```python
from build123d import *

# Parameters (mm, degrees)
F1_DEPTH = 1587.5
F2_R     = 3.175
F3_DEPTH = 25.401
F4_W     = 25.4
F4_H     = 393.7
F5_DEPTH = 3.175


with BuildPart() as f1:
    # F0 (on Top) → F1 (new body)
    with BuildSketch(Plane.XY):
        Polygon((25.4, 196.85), (0, 196.85), (0, -196.85), (25.4, -196.85), (25.4, -193.675), (3.175, -193.675), (3.175, 193.675), (25.4, 193.675), align=None)
    extrude(amount=F1_DEPTH)

    # F2 (on face) → F3 (cut, through all)
    with BuildSketch(Plane(origin=(0, 0, 0), x_dir=(0, -1, 0), z_dir=(-1, 0, 0))):
        with BuildLine():
            Line((184.15, 793.75), (190.5, 793.75))
            ThreePointArc((190.5, 793.75), (187.325, 796.925), (184.15, 793.75))
        make_face()
        with BuildLine():
            ThreePointArc((-193.675, 793.75), (-190.5, 790.575), (-187.325, 793.75))
            Line((-187.325, 793.75), (-193.675, 793.75))
        make_face()
        with BuildLine():
            Line((-193.675, 793.75), (-187.325, 793.75))
            ThreePointArc((-187.325, 793.75), (-190.5, 796.925), (-193.675, 793.75))
        make_face()
        with BuildLine():
            ThreePointArc((184.15, 793.75), (187.325, 790.575), (190.5, 793.75))
            Line((190.5, 793.75), (184.15, 793.75))
        make_face()
        with Locations((187.325, 844.55)):
            Circle(F2_R)
        with Locations((187.325, 895.35)):
            Circle(F2_R)
        with Locations((187.325, 946.15)):
            Circle(F2_R)
        with Locations((187.325, 996.95)):
            Circle(F2_R)
        with Locations((187.325, 1047.75)):
            Circle(F2_R)
        with Locations((187.325, 1098.55)):
            Circle(F2_R)
        with Locations((187.325, 1149.35)):
            Circle(F2_R)
        with Locations((187.325, 1200.15)):
            Circle(F2_R)
        with Locations((187.325, 1250.95)):
            Circle(F2_R)
        with Locations((187.325, 1301.75)):
            Circle(F2_R)
        with Locations((187.325, 1352.55)):
            Circle(F2_R)
        with Locations((187.325, 1403.35)):
            Circle(F2_R)
        with Locations((187.325, 1454.15)):
            Circle(F2_R)
        with Locations((187.325, 1504.95)):
            Circle(F2_R)
        with Locations((-190.5, 844.55)):
            Circle(F2_R)
        with Locations((-190.5, 895.35)):
            Circle(F2_R)
        with Locations((-190.5, 946.15)):
            Circle(F2_R)
        with Locations((-190.5, 996.95)):
            Circle(F2_R)
        with Locations((-190.5, 1047.75)):
            Circle(F2_R)
        with Locations((-190.5, 1098.55)):
            Circle(F2_R)
        with Locations((-190.5, 1149.35)):
            Circle(F2_R)
        with Locations((-190.5, 1200.15)):
            Circle(F2_R)
        with Locations((-190.5, 1250.95)):
            Circle(F2_R)
        with Locations((-190.5, 1301.75)):
            Circle(F2_R)
        with Locations((-190.5, 1352.55)):
            Circle(F2_R)
        with Locations((-190.5, 1403.35)):
            Circle(F2_R)
        with Locations((-190.5, 1454.15)):
            Circle(F2_R)
        with Locations((-190.5, 1504.95)):
            Circle(F2_R)
        with Locations((187.325, 742.95)):
            Circle(F2_R)
        with Locations((187.325, 692.15)):
            Circle(F2_R)
        with Locations((187.325, 641.35)):
            Circle(F2_R)
        with Locations((187.325, 590.55)):
            Circle(F2_R)
        with Locations((187.325, 539.75)):
            Circle(F2_R)
        with Locations((187.325, 488.95)):
            Circle(F2_R)
        with Locations((187.325, 438.15)):
            Circle(F2_R)
        with Locations((187.325, 387.35)):
            Circle(F2_R)
        with Locations((187.325, 336.55)):
            Circle(F2_R)
        with Locations((187.325, 285.75)):
            Circle(F2_R)
        with Locations((187.325, 234.95)):
            Circle(F2_R)
        with Locations((187.325, 184.15)):
            Circle(F2_R)
        with Locations((187.325, 133.35)):
            Circle(F2_R)
        with Locations((187.325, 82.55)):
            Circle(F2_R)
        with Locations((-190.5, 742.95)):
            Circle(F2_R)
        with Locations((-190.5, 692.15)):
            Circle(F2_R)
        with Locations((-190.5, 641.35)):
            Circle(F2_R)
        with Locations((-190.5, 590.55)):
            Circle(F2_R)
        with Locations((-190.5, 539.75)):
            Circle(F2_R)
        with Locations((-190.5, 488.95)):
            Circle(F2_R)
        with Locations((-190.5, 438.15)):
            Circle(F2_R)
        with Locations((-190.5, 387.35)):
            Circle(F2_R)
        with Locations((-190.5, 336.55)):
            Circle(F2_R)
        with Locations((-190.5, 285.75)):
            Circle(F2_R)
        with Locations((-190.5, 234.95)):
            Circle(F2_R)
        with Locations((-190.5, 184.15)):
            Circle(F2_R)
        with Locations((-190.5, 133.35)):
            Circle(F2_R)
        with Locations((-190.5, 82.55)):
            Circle(F2_R)
        with Locations((187.325, 31.75)):
            Circle(F2_R)
        with Locations((-190.5, 31.75)):
            Circle(F2_R)
        with Locations((187.325, 1555.75)):
            Circle(F2_R)
        with Locations((-190.5, 1555.75)):
            Circle(F2_R)
    extrude(amount=-F3_DEPTH, mode=Mode.SUBTRACT)

    # F4 (on face) → F5 (join)
    with BuildSketch(Plane(origin=(0, 0, 0), x_dir=(1, 0, 0), z_dir=(0, 0, -1))):
        with Locations((12.7, 0)):
            Rectangle(F4_W, F4_H)
    extrude(amount=F5_DEPTH)


solid = f1.part
```
The listing builds one solid part. Answer for the finished solid, in the listing's coordinates (mm). Round coordinates to 2 decimals unless told otherwise and drop trailing zeros. Loops run counter-clockwise (first coordinate to the right, second up) from the corner with the lowest first, then second, coordinate; pieces in that order, holes last.
1) Consider line 1 (Y direction, x = 2.2, z = 539.75) (3 decimals); line 2 (Y direction, x = 19.25, z = 1281.5) (3 decimals); line 3 (X direction, y = -5.5, z = 874) (3 decimals). Determine where each line is inside the solid, lowest interval first.
Outcome:
line 1: y = -196.85 to -190.5, -184.15 to 187.325, 193.675 to 196.85
line 2: y = -196.85 to -193.675, 193.675 to 196.85
line 3: x = 0 to 3.175
2) Given P1, Ø8.5, axis at y = -187.325, z = 234.95, coming from the +X side (3 decimals); P2, Ø4, axis at y = 190.5, z = 387.35, coming from the -X side; P3, Ø8.5, axis at y = 190.5, z = 844.55, coming from the +X side, each flat-ended and moving along its own axis, determine where each tip first touches the part or whether it passes through.
Outcome:
P1: stops at x = 3.175
P2: passes through
P3: stops at x = 25.4
3) A cutting plane is placed at B-B on x = 8. Determine the outline of the cut face in (y, z) (3 decimals), plus the area to 3 significant figures.
Outcome:
outline: (-196.85, -3.175) - (196.85, -3.175) - (196.85, 1587.5) - (193.675, 1587.5) - (193.675, 0) - (-193.675, 0) - (-193.675, 1587.5) - (-196.85, 1587.5) - close
area: 11,300 mm2
4) A cutting plane is placed at C-C on y = -24. Determine the outline of the cut face in (x, z) (3 decimals).
Outcome:
outline: (0, -3.175) - (25.4, -3.175) - (25.4, 0) - (3.175, 0) - (3.175, 1587.5) - (0, 1587.5) - close
5) For a pull along Y with two mould halves and no side action, classify faces 1 (the face through (13, -3, -3.175)), 2 (the face through (3.175, -3, 783)), 3 (the face through (13, 196.85, 803)), 4 (the face through (13, -196.85, 803)) as released by +Y, released by -Y, zero draft, split by the parting line, or undercut.
Outcome:
face 1: zero draft
face 2: undercut
face 3: released by +Y
face 4: released by -Y
6) A cutting plane is placed at A-A on z = 150.5. Determine the outline of the cut face in (x, y) (3 decimals), plus the area to 3 significant figures.
Outcome:
outline: (0, -196.85) - (25.4, -196.85) - (25.4, -193.675) - (3.175, -193.675) - (3.175, 193.675) - (25.4, 193.675) - (25.4, 196.85) - (0, 196.85) - close
area: 1,390 mm2
